Geometry check sheet. Reference: the model listing, model coordinates, mm. Face numbers are marked on the shaded views. Coordinates: 2 decimals unless noted, no trailing zeros. Loops run counter-clockwise (first coordinate to the right, second up) from the corner with the lowest first, then second, coordinate; pieces in that order, holes last. Notation, with made-up numbers: (75.25, 59.25) -> (95.25, 59.25) arc R29 cw to (95.25, 80.25) -> close; hole circle Ø10 at (79.5, 50.5). An arc over 180 degrees is marked (long way). Answer as a JSON object with one key per item and string values.
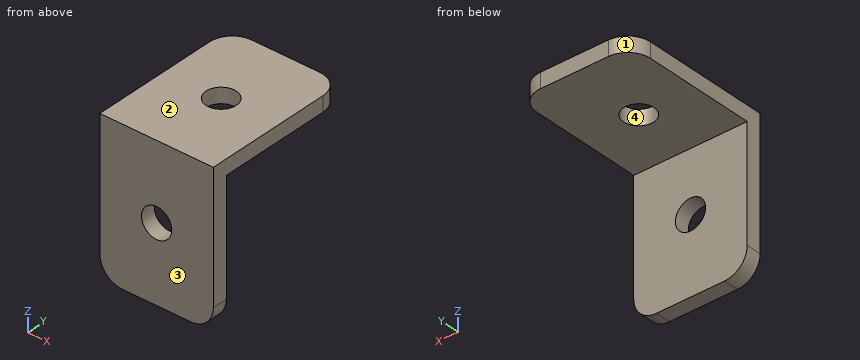
from build123d import *

# Parameters (mm, degrees)
SKETCH1_R           = 2
BOSS_EXTRUDE1_DEPTH = 2
SKETCH2_R           = 2
SKETCH2_W           = 15
SKETCH2_H           = 2
BOSS_EXTRUDE2_DEPTH = 2


with BuildPart() as part:
    # Sketch1 → Boss-Extrude1 (new body)
    with BuildSketch(Plane(origin=(0, 0, 0), x_dir=(1, 0, 0), z_dir=(0, 1, 0))):
        with BuildLine():
            Line((0, 0), (0, 15))
            ThreePointArc((0, 15), (0.878679656, 17.121320344), (3, 18))
            Line((3, 18), (12, 18))
            ThreePointArc((12, 18), (14.121320344, 17.121320344), (15, 15))
            Line((15, 15), (15, 0))
            Line((15, 0), (0, 0))
        make_face()
        with Locations((7.5, 8)):
            Circle(SKETCH1_R, mode=Mode.SUBTRACT)
    extrude(amount=BOSS_EXTRUDE1_DEPTH)

    # Sketch2 → Boss-Extrude2 (add)
    with BuildSketch(Plane.XY):
        with BuildLine():
            Line((0, 17), (0, 2))
            Line((0, 2), (15, 2))
            Line((15, 2), (15, 17))
            ThreePointArc((15, 17), (14.121320344, 19.121320344), (12, 20))
            Line((12, 20), (3, 20))
            ThreePointArc((3, 20), (0.878679656, 19.121320344), (0, 17))
        make_face()
        with Locations((7.5, 10)):
            Circle(SKETCH2_R, mode=Mode.SUBTRACT)
        with Locations((7.5, 1)):
            Rectangle(SKETCH2_W, SKETCH2_H)
    extrude(amount=BOSS_EXTRUDE2_DEPTH)


solid = part.part
1. Depth check by flat-ended pin: P1, Ø1, axis at x = 6, y = 7, coming from the -Z side; P2, Ø4.5, axis at x = 6, z = -12, coming from the +Y side. Enter the tip coordinate at first touch or a pass-through.
Evaluation:
{"P1": "stops at z = 0", "P2": "stops at y = 2"}
2. Mould release check, pull along Y, two halves, no side actions. Record for the marked faces 1, 2, 3 and 4: released by +Y, released by -Y, zero draft, split by the parting line, or undercut.
Evaluation:
{"face 1": "released by +Y", "face 2": "zero draft", "face 3": "released by -Y", "face 4": "undercut"}
3. Section check A-A, the plane z = -8. Record the boundary of the cut face in (x, y).
Evaluation:
{"outline": "(0, 0) -> (5.5, 0) -> (5.5, 2) -> (0, 2) -> close; (9.5, 0) -> (15, 0) -> (15, 2) -> (9.5, 2) -> close"}
4. Section check B-B, the plane x = 7.5. Record the boundary of the cut face in (y, z), then the cut area to 3 significant figures.
Evaluation:
{"outline": "(0, -18) -> (2, -18) -> (2, -10) -> (0, -10) -> close; (0, -6) -> (2, -6) -> (2, 0) -> (8, 0) -> (8, 2) -> (0, 2) -> close; (12, 0) -> (20, 0) -> (20, 2) -> (12, 2) -> close", "area": "60.0 mm^2"}
5. Section check D-D, the plane x = 5. Record the boundary of the cut face in (y, z), then the cut area to 3 significant figures.
Evaluation:
{"outline": "(0, -18) -> (2, -18) -> (2, 0) -> (20, 0) -> (20, 2) -> (0, 2) -> close", "area": "76.0 mm^2"}
6. Thickness scan on probe 1 along X at (y, z) = (1.55, -8); probe 2 along Z at (x, y) = (7.5, 1.65); probe 3 along Y at (x, z) = (13.75, -4.25). Record the ranges inside material, lowest first. Write a range as from..to.
Evaluation:
{"probe 1": "x = 0..5.5, 9.5..15", "probe 2": "z = -18..-10, -6..2", "probe 3": "y = 0..2"}
